Can you work these out from the drawing? Everything is in mm from the part's minimum corner. A direction names the side the tool comes from. Round coordinates to 2 decimals unless told otherwise and drop trailing zeros. Loops run counter-clockwise (first coordinate to the right, second up) from the corner with the lowest first, then second, coordinate; pieces in that order, holes last. Notation, with made-up numbers: M -30,83.25 L 20,83.25 A29 ccw 20,113.25 Z; hole C 61.25,48.5 d2. An arc over 180 degrees is marked long. Use a Markdown table: item, result.
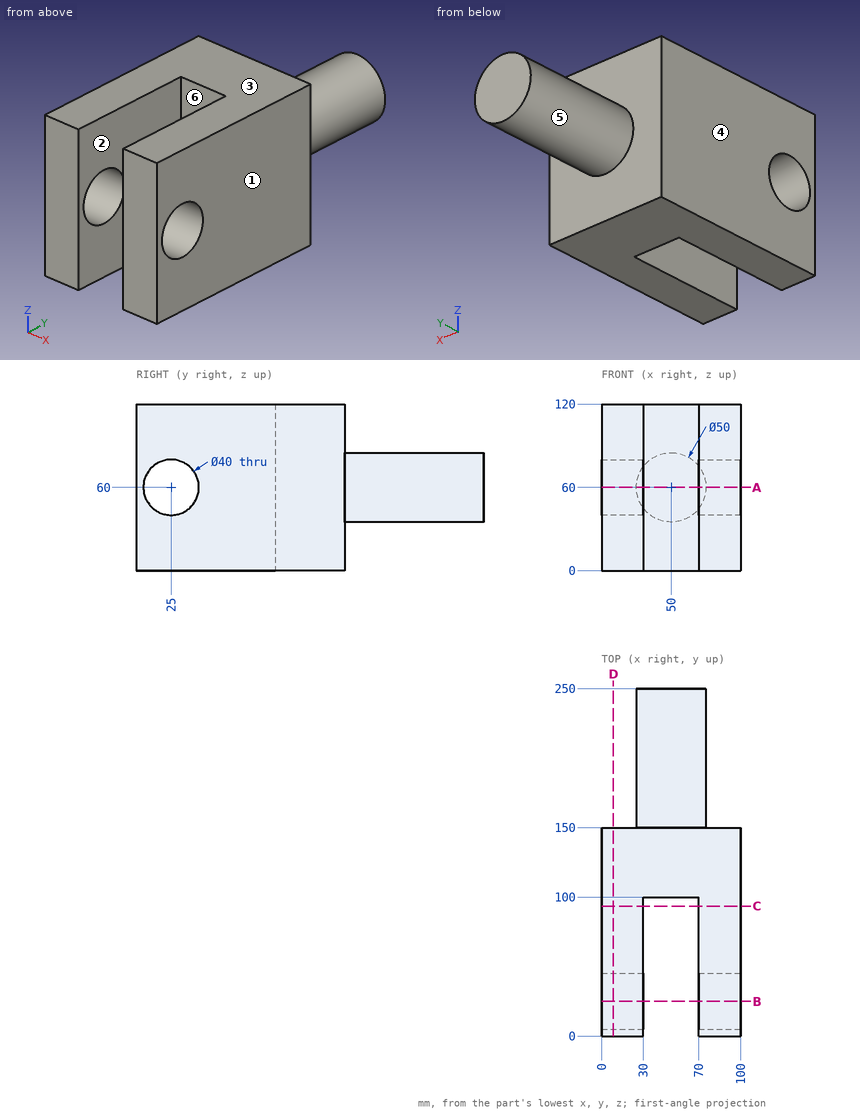
1. Imagine slicing it at D-D, the plane x = 8.5. Write out the boundary of the cut face in (y, z), then the cut area to 3 significant figures.
Answer sheet:
| item | result |
|---|---|
| outline | M 0,0 L 150,0 L 150,120 L 0,120 Z; hole C 25,60 d40 |
| area | 16,700 mm2 |
2. We'd pull the mould along X, two halves only. Please class the marked faces 3, 4, 5 and 6: +X half, -X half, draft (parallel to the pull), parting line (faces both ways), or undercut.
Answer sheet:
| item | result |
|---|---|
| face 3 | draft |
| face 4 | -X half |
| face 5 | parting line |
| face 6 | undercut |
3. For pin 1 Ø12 at (x, z) = (51, 89.5) entering from -Y; pin 2 Ø6 at (y, z) = (194.5, 85.5) entering from -X; pin 3 Ø12 at (y, z) = (163.5, 60.5) entering from -X, each with a flat end and sliding along its axis, tell me the tip position at first contact or that it passes through.
Answer sheet:
| item | result |
|---|---|
| pin 1 | y = 100 |
| pin 2 | x = 39.1 |
| pin 3 | x = 25 |
4. Imagine slicing it at B-B, the plane y = 25. Write out the boundary of the cut face in (x, z).
Answer sheet:
| item | result |
|---|---|
| outline | M 0,0 L 30,0 L 30,40 L 0,40 Z; M 0,80 L 30,80 L 30,120 L 0,120 Z; M 70,0 L 100,0 L 100,40 L 70,40 Z; M 70,80 L 100,80 L 100,120 L 70,120 Z |
5. Imagine slicing it at A-A, the plane z = 60. Write out the boundary of the cut face in (x, y).
Answer sheet:
| item | result |
|---|---|
| outline | M 0,0 L 30,0 L 30,5 L 0,5 Z; M 0,45 L 30,45 L 30,100 L 70,100 L 70,45 L 100,45 L 100,150 L 75,150 L 75,250 L 25,250 L 25,150 L 0,150 Z; M 70,0 L 100,0 L 100,5 L 70,5 Z |
6. Which directions (+Z, -Z, +X, -X, +Y, -Y) give clear straight access to the entire face, cutting with the end or side of a thin tool? Please do the marked faces 1 and 2.
Answer sheet:
| item | result |
|---|---|
| face 1 | +Z, -Z, +X, +Y, -Y |
| face 2 | +Z, -Z, -Y |
7. Imagine slicing it at C-C, the plane y = 93.5. Write out the boundary of the cut face in (x, z), then the cut area to 3 significant figures.
Answer sheet:
| item | result |
|---|---|
| outline | M 0,0 L 30,0 L 30,120 L 0,120 Z; M 70,0 L 100,0 L 100,120 L 70,120 Z |
| area | 7,200 mm2 |
8. I need wall thicknesses on probe 1 along Y at (x, z) = (20, 60); probe 2 along X at (y, z) = (61, 46.5); probe 3 along Y at (x, z) = (23, 87). Which ranges of each line are inside material? Lowest first, please. Write a range as from..to.
Answer sheet:
| item | result |
|---|---|
| probe 1 | 0..5, 45..150 |
| probe 2 | 0..30, 70..100 |
| probe 3 | 0..150 |
